Autodesk Inventor part; units mm, degrees
ref_plane "YZ Plane" through (0, 0, 0) normal (1, 0, 0) x (0, 1, 0)
ref_plane "XZ Plane" through (0, 0, 0) normal (0, 1, 0) x (-1, 0, 0)
ref_plane "XY Plane" through (0, 0, 0) normal (0, 0, 1) x (1, 0, 0)
sketch "Sketch1" plane through (0, 0, 0) normal (0, 0, 1) x (1, 0, 0)
  line L0 (-7.3323, 12.7) -> (7.3323, 12.7)
  line L1 (7.3323, 12.7) -> (14.6647, 0)
  line L2 (14.6647, 0) -> (7.3323, -12.7)
  line L3 (7.3323, -12.7) -> (-7.3323, -12.7)
  line L4 (-7.3323, -12.7) -> (-14.6647, 0)
  line L5 (-14.6647, 0) -> (-7.3323, 12.7)
  circle A0 centre (0, 0) radius 9.525
  dimension "d0" = 25.4
  dimension "d1" = 19.05
extrude "Extrusion1" add sketch "Sketch1" along normal mid plane 7.9502
chamfer "Chamfer1" distance 0.127 angle 45 2 edges at (-9.525, 0, 3.9751) (-9.525, 0, -3.9751)
sketch "Sketch2" plane through (0, 0, 0) normal (0, 1, 0) x (-1, 0, 0)
  line L0 (11.8999, 3.9751) -> (14.6647, 3.2343)
  line L1 (14.6647, 3.2343) -> (14.6647, 3.9751)
  line L2 (14.6647, 3.9751) -> (11.8999, 3.9751)
  line L3 (14.6647, 3.9751) -> (7.3323, 3.9751) construction
  line L4 (7.3323, 3.9751) -> (7.3323, -3.9751) construction
  line L5 (14.6647, 3.9751) -> (7.3323, 3.9751) construction
  line L6 (14.6647, 3.9751) -> (14.6647, -3.9751) construction
  line L7 (7.3323, -3.9751) -> (14.6647, -3.9751) construction
  line L8 (0, 0) -> (14.6647, 0) construction
  line L9 (11.8999, -3.9751) -> (14.6647, -3.2343)
  line L10 (14.6647, -3.2343) -> (14.6647, -3.9751)
  line L11 (14.6647, -3.9751) -> (11.8999, -3.9751)
  line L12 (0, -3.8938) -> (0, 3.8938)
  dimension "d7" = 11.8999
  dimension "d8" = 15
revolve "Revolution1" cut sketch "Sketch2" angle 360 about axis through (0, 0, -10) along (0, 0, 1)
thread "Thread1"
equation "\"d0\" = AN924_A"
equation "\"d1\" = AN924_T"
equation "\"d2\" = AN924_B"
equation "\"d7\" = 0.5 * AN924_G"
equation "\"AN924_A\" = 25.4"
equation "\"AN924_B\" = 7.9502"
equation "\"AN924_G\" = 23.7998"
equation "\"AN924_T\" = 19.05"
equation "\"Tube_OD\" = 12.7"
properties part number "AN924-8D" material "Aluminum 2014-T6"
Build history of the part. All positions in model axes, mm. Give positions to 0.01 mm unless a question says otherwise; leave off trailing zeros. Order: outer loops, then holes, each group sorted by start corner. A loop starts at its lowest first (then second) coordinate and runs counter-clockwise, first axis right, second up. Notation, with made-up numbers: M -20.5,59.25 L 1.5,59.25 A20 cw 1.5,95.25 Z; hole C 77,-38 d7. An arc over 180 degrees is marked long. Write item = value, one per line. Start each with the question number.
(1) Slice it at A-A on x = 0. Write the cut outline in (y, z) (3 decimals).
(2) Pin check, flat tip, straight feed: pin 1 Ø2 at (x, z) = (11.5, 2.5) entering from +Y. Stop position of the tip, or through.
(3) Probe L1, parallel to Y at x = 0, z = 2.25 (3 decimals); L2, parallel to X at y = -3, z = 1.5; L3, parallel to X at y = -5, z = 0.5. List the from-to ranges inside material, lowest first. Write a range as [from, to].
(4) Slice it at B-B on z = 1.5. Write the cut outline in (x, y) (3 decimals), plus the area to 3 significant figures.
(5) Two-plate mould, pull along Y, no slides. Class faces 1 (the flat face through (0, 10, -3.975)), 2 (the conical face through (-11.15, 4.62, -3.93)), 3 (the cylindrical face through (-7.559, 5.796, -0.054)), 4 (the flat face through (0, 12.7, 0)): released by +Y, released by -Y, zero draft, split by the parting line, or undercut.
Responses:
q1.outline = M -12.7,-3.761 L -11.9,-3.975 L -9.652,-3.975 L -9.525,-3.848 L -9.525,3.848 L -9.652,3.975 L -11.9,3.975 L -12.7,3.761 Z; M 9.525,-3.848 L 9.652,-3.975 L 11.9,-3.975 L 12.7,-3.761 L 12.7,3.761 L 11.9,3.975 L 9.652,3.975 L 9.525,3.848 Z
q2.pin_1 = 7.21
q3.L1 = [-12.7, -9.525], [9.525, 12.7]
q3.L2 = [-12.93, -9.04], [9.04, 12.93]
q3.L3 = [-11.78, -8.11], [8.11, 11.78]
q4.outline = M -14.665,0 L -7.332,-12.7 L 7.332,-12.7 L 14.665,0 L 7.332,12.7 L -7.332,12.7 Z; hole C 0,0 d19.05
q4.area = 274 mm2
q5.face_1 = zero draft
q5.face_2 = split by the parting line
q5.face_3 = undercut
q5.face_4 = released by +Y
